Input: part model. Units: mm. Frame: model coordinates. A direction names the side the tool comes from. Round coordinates to 2 decimals unless told otherwise and drop trailing zeros. Loops run counter-clockwise (first coordinate to the right, second up) from the corner with the lowest first, then second, coordinate; pieces in that order, holes last. Notation, with made-up numbers: (44, 79.5) -> (66, 79.5) arc R14 ccw to (66, 100.5) -> close; hole circle Ø5 at (-15, -8). An arc over 180 degrees is marked (long way). One line per question, with ' | ' between items. Start each with the question number.
Q1. Material intervals for L1, parallel to Y at x = 5, z = 45.5; L2, parallel to X at y = -11, z = -45; L3, parallel to X at y = -33, z = -3.5, sorted ascending.
Q2. Cut plane D-D on z = 1. Return loops of the section in (x, y), and give its area (3 significant figures).
Q3. Cut plane B-B on y = -34. Return loops of the section in (x, z), and give its area (3 significant figures).
Q4. Mould query, pull axis Z, two halves, no side actions, for faces 5 (the face through (-8, 0, -4)), 6 (the face through (4, -29, -54.635)), 7 (the face through (-7, -30, -1)), 8 (the face through (4, -32, 45.02)). Classes: pulls with the +Z half, pulls with the -Z half, needs draft (parallel to the pull), parting line crosses it, or undercut.
Q5. Cut plane C-C on x = -20.5. Return loops of the section in (y, z), and give its area (4 significant figures).
Q6. Cut plane A-A on x = -0.5. Return loops of the section in (y, z).
Q7. Access query for faces 1 (the face through (-1, -9.177, -57)), 2 (the face through (0.244, -48.023, -57.17)), 3 (the face through (-1, -11.562, 48)), 4 (the face through (-1, -6, 50.02)). Directions: +Z, -Z, +X, -X, +Y, -Y. A direction counts if a zero-diameter tool reaches every point of the face in a straight line with its end or side. Return the directions, or none.
Q8. Contact query for flat-ended pins moving along their axis: P1, Ø12.5, axis at x = -5, y = -28, coming from the +Z side; P2, Ø21.5, axis at y = -32.5, z = 7.5, coming from the -X side; P3, Ø1.5, axis at y = -21.5, z = -5, coming from the +X side. Output: stop coordinate, or through.
from build123d import *

# Parameters (mm, degrees)
F0_W     = 67.0811040951
F0_H     = 109.6547991037
F1_DEPTH = 60
F2_R     = 40.3328803273
F3_DEPTH = 60
F4_W     = 67.0811040951
F4_H     = 40.9807842225
F5_DEPTH = 5
F7_DEPTH = 5
F9_DEPTH = 10


with BuildPart() as f1:
    # F0 (on Front) → F1 (new body)
    with BuildSketch(Plane.XZ):
        with Locations((-0.2257995927, -4.8074126244)):
            Rectangle(F0_W, F0_H)
    extrude(amount=F1_DEPTH)

    # F2 (on face) → F3 (cut)
    with BuildSketch(Plane.XZ.offset(60)):
        with Locations((33.3147524549, -2.237562323)):
            Circle(F2_R)
    extrude(amount=-F3_DEPTH, mode=Mode.SUBTRACT)

    # F4 (on face) → F5 (cut)
    with BuildSketch(Plane.XY.offset(50.0199869275)):
        with Locations((-0.2257995927, -32.0525960997)):
            Rectangle(F4_W, F4_H)
    extrude(amount=-F5_DEPTH, mode=Mode.SUBTRACT)

    # F6 (on face) → F7 (cut)
    with BuildSketch(Plane(origin=(0, 0, -59.6348121762), x_dir=(1, 0, 0), z_dir=(0, 0, -1))):
        Polygon((-33.7663516402, 49.7098267078), (-33.7663516402, 9.1774007306), (33.3147524549, 9.1774007306), (33.3147524549, 46.3831014931), align=None)
    extrude(amount=-F7_DEPTH, mode=Mode.SUBTRACT)

    # F8 (on face) → F9 (cut)
    with BuildSketch(Plane(origin=(-33.7663516402, 0, 0), x_dir=(0, -1, 0), z_dir=(-1, 0, 0))):
        Polygon((52.5429882109, 45.0199869275), (11.5622039884, 45.0199869275), (9.1774007306, -54.6348121762), (49.7098267078, -54.6348121762), align=None)
    extrude(amount=-F9_DEPTH, mode=Mode.SUBTRACT)


solid = f1.part
Results:
1) L1: -60 to -52.54, -11.56 to 0 | L2: -23.77 to 33.31 | L3: -23.77 to -7
2) outline: (-33.77, -60) -> (-6.89, -60) -> (-6.89, 0) -> (-33.77, 0) -> (-33.77, -10.51) -> (-23.77, -10.51) -> (-23.77, -51.29) -> (-33.77, -51.29) -> close | area: 1,200 mm^2
3) outline: (-23.77, -54.63) -> (33.31, -54.63) -> (33.31, -42.57) arc R40.33 cw to (33.31, 38.1) -> (33.31, 45.02) -> (-23.77, 45.02) -> close | area: 3,130 mm^2
4) face 5: needs draft | face 6: pulls with the -Z half | face 7: undercut | face 8: pulls with the +Z half
5) outline: (-60, -59.63) -> (-49.05, -59.63) -> (-49.05, -54.63) -> (-9.18, -54.63) -> (-9.18, -59.63) -> (0, -59.63) -> (0, 50.02) -> (-11.56, 50.02) -> (-11.56, 45.02) -> (-52.54, 45.02) -> (-52.54, 50.02) -> (-60, 50.02) -> close | area: 6,175 mm^2
6) outline: (-60, -59.63) -> (-48.06, -59.63) -> (-48.06, -54.63) -> (-9.18, -54.63) -> (-9.18, -59.63) -> (0, -59.63) -> (0, -24.22) -> (-60, -24.22) -> close; (-60, 19.75) -> (0, 19.75) -> (0, 50.02) -> (-11.56, 50.02) -> (-11.56, 45.02) -> (-52.54, 45.02) -> (-52.54, 50.02) -> (-60, 50.02) -> close
7) face 1: -Z, +X, -X | face 2: -Z, -X | face 3: +Z, +X, -X | face 4: +Z, +X, -X, +Y, -Y
8) P1: z = 45.02 | P2: x = -23.77 | P3: x = -6.86
